Here's the drawing with two shaded views (mm, measured from the low corner). I have some questions. A direction names the side the tool comes from. Give positions to 0.01 mm unless a question says otherwise; leave off trailing zeros. Loops run counter-clockwise (first coordinate to the right, second up) from the corner with the lowest first, then second, coordinate; pieces in that order, holes last. Notation, with made-up numbers: (29.5, 13) - (52.5, 13) arc R19 ccw to (52.5, 37) - close; hole circle Ø3 at (19.25, 32.5). An arc over 180 degrees is marked (long way). Use one line per item in the form item = value.
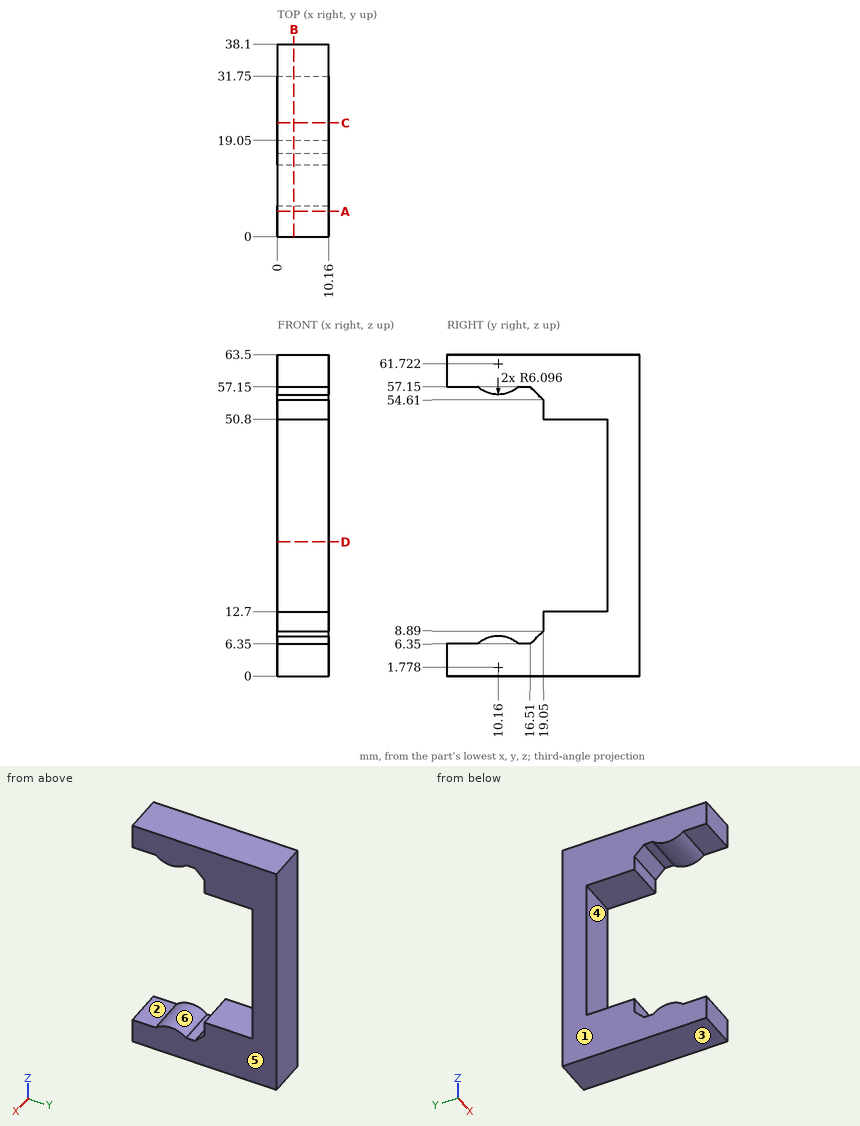
(1) For the marked faces 4, 5 and 6, which set-ups out of +Z, -Z, +X, -X, +Y, -Y let a thin tool reach every point of the face, with its end or its side?
Geometry says:
face_4 = +X, -X, -Y
face_5 = +Z, -Z, +X, +Y, -Y
face_6 = +X, -X
(2) If we section it at C-C (y = 22.5): List the corners of the cut face in (x, z) for me, plus the area to 3 significant figures.
Geometry says:
outline = (0, 0) - (10.16, 0) - (10.16, 12.7) - (0, 12.7) - close; (0, 50.8) - (10.16, 50.8) - (10.16, 63.5) - (0, 63.5) - close
area = 258 mm²
(3) If we section it at A-A (y = 5): List the corners of the cut face in (x, z) for me.
Geometry says:
outline = (0, 0) - (10.16, 0) - (10.16, 6.35) - (0, 6.35) - close; (0, 57.15) - (10.16, 57.15) - (10.16, 63.5) - (0, 63.5) - close
(4) Thinking about a two-plate mould opening in Z: for the marked faces 1, 2 and 3, which applies, pulls with the +Z half, pulls with the -Z half, needs draft (parallel to the pull), parting line crosses it, or undercut?
Geometry says:
face_1 = needs draft
face_2 = undercut
face_3 = pulls with the -Z half
(5) For P1, Ø5, axis at x = 4.5, y = 2.5, coming from the -Z side; P2, Ø4, axis at x = 4, z = 11.5, coming from the -Y side; P3, Ø3, axis at x = 7.5, z = 34, coming from the -Y side; P4, Ø1.9, axis at x = 6.5, z = 52, coming from the -Y side, each with a flat end and sliding along its axis, tell me the tip position at first contact or that it passes through.
Geometry says:
P1 = 0
P2 = 19.05
P3 = 31.75
P4 = 19.05
(6) If I drill on probe 1 along Z at (x, y) = (2.75, 21); probe 2 along Z at (x, y) = (7.5, 2.5); probe 3 along Y at (x, z) = (8.25, 13), over which ranges is the centre line in solid material (lowest first)?
Geometry says:
probe_1 = 0 to 12.7, 50.8 to 63.5
probe_2 = 0 to 6.35, 57.15 to 63.5
probe_3 = 31.75 to 38.1
(7) If we section it at B-B (x = 3.25): List the corners of the cut face in (y, z) for me.
Geometry says:
outline = (0, 0) - (38.1, 0) - (38.1, 63.5) - (0, 63.5) - (0, 57.15) - (6.13, 57.15) arc R6.1 ccw to (14.19, 57.15) - (16.51, 57.15) - (19.05, 54.61) - (19.05, 50.8) - (31.75, 50.8) - (31.75, 12.7) - (19.05, 12.7) - (19.05, 8.89) - (16.51, 6.35) - (14.19, 6.35) arc R6.1 ccw to (6.13, 6.35) - (0, 6.35) - close
(8) If we section it at D-D (z = 26.5): List the corners of the cut face in (x, y) for me, plus the area to 3 significant figures.
Geometry says:
outline = (0, 31.75) - (10.16, 31.75) - (10.16, 38.1) - (0, 38.1) - close
area = 64.5 mm²
